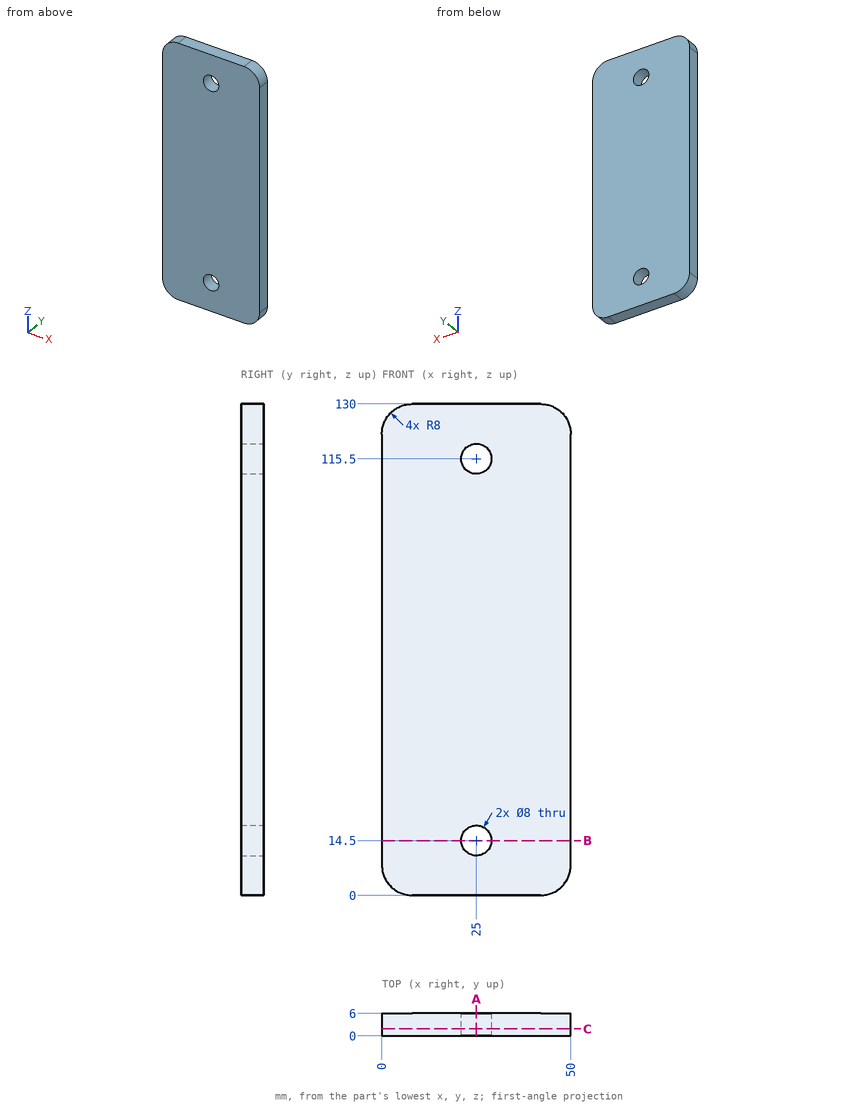
Source: three-view drawing plus pictorial views. Frame: mm from the lowest corner of the part. Coordinates: 2 decimals unless noted, no trailing zeros. Loops run counter-clockwise (first coordinate to the right, second up) from the corner with the lowest first, then second, coordinate; pieces in that order, holes last. Notation, with made-up numbers: (68, -35) - (82, -35) arc R16 ccw to (82, -30) - close; hole circle Ø6 at (-39, 85.5). An arc over 180 degrees is marked (long way). One line per item, written item: value. Start each with the question number.
1. Ray query, L1, parallel to Z at x = 25, y = 3.3; L2, parallel to X at y = 2.5, z = 14.5; L3, parallel to Z at x = 27.5, y = 1.9. Return the intervals inside material, ascending.
2. Section C-C (y = 1.9). Return the cut outline in (x, z).
3. Section A-A (x = 25). Return the cut outline in (y, z), and give its area (3 significant figures).
4. Section B-B (z = 14.5). Return the cut outline in (x, y), and give its area (3 significant figures).
Verdict:
1. L1: z = 0 to 10.5, 18.5 to 111.5, 119.5 to 130
1. L2: x = 0 to 21, 29 to 50
1. L3: z = 0 to 11.38, 17.62 to 112.38, 118.62 to 130
2. outline: (0, 8) arc R8 ccw to (8, 0) - (42, 0) arc R8 ccw to (50, 8) - (50, 122) arc R8 ccw to (42, 130) - (8, 130) arc R8 ccw to (0, 122) - close; hole circle Ø8 at (25, 14.5); hole circle Ø8 at (25, 115.5)
3. outline: (0, 0) - (6, 0) - (6, 10.5) - (0, 10.5) - close; (0, 18.5) - (6, 18.5) - (6, 111.5) - (0, 111.5) - close; (0, 119.5) - (6, 119.5) - (6, 130) - (0, 130) - close
3. area: 684 mm2
4. outline: (0, 0) - (21, 0) - (21, 6) - (0, 6) - close; (29, 0) - (50, 0) - (50, 6) - (29, 6) - close
4. area: 252 mm2
